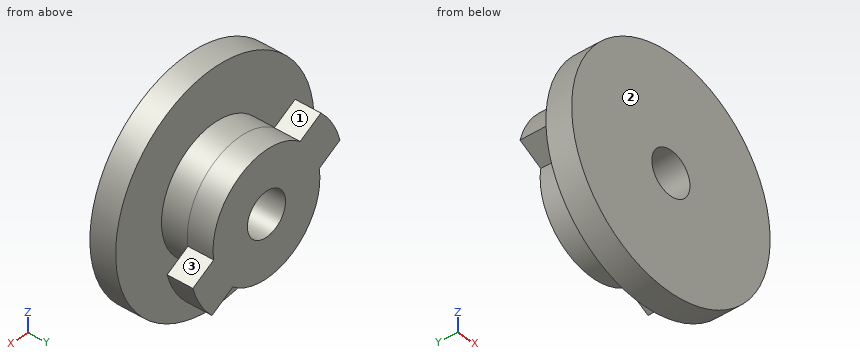
from build123d import *

# Parameters (mm, degrees)
BOSS_EXTRUDE1_DEPTH = 3
BOSS_EXTRUDE2_START = 3
SKETCH2_R           = 7
BOSS_EXTRUDE2_DEPTH = 3
SKETCH3_R           = 13
BOSS_EXTRUDE3_DEPTH = 3
SKETCH4_R           = 2.5
CUT_EXTRUDE1_DEPTH  = 20


with BuildPart() as part:
    # Sketch1 → Boss-Extrude1 (new body)
    with BuildSketch(Plane(origin=(0, 0, 0), x_dir=(-1, 0, 0), z_dir=(0, 1, 0))):
        with BuildLine():
            Line((4.412375826, -57.65977305), (7.135254916, -56.087718075))
            ThreePointArc((7.135254916, -56.087718075), (8.660254038, -58.094010768), (9.635254916, -60.417845094))
            Line((9.635254916, -60.417845094), (6.912375826, -61.989900069))
            ThreePointArc((6.912375826, -61.989900069), (3.5, -69.156188594), (-4.412375826, -68.528248485))
            Line((-4.412375826, -68.528248485), (-7.135254916, -70.10030346))
            ThreePointArc((-7.135254916, -70.10030346), (-8.660254038, -68.094010768), (-9.635254916, -65.770176441))
            Line((-9.635254916, -65.770176441), (-6.912375826, -64.198121466))
            ThreePointArc((-6.912375826, -64.198121466), (-3.5, -57.031832941), (4.412375826, -57.65977305))
        make_face()
    extrude(amount=BOSS_EXTRUDE1_DEPTH)

    # Sketch2 → Boss-Extrude2 (add)
    with BuildSketch(Plane.XZ.offset(BOSS_EXTRUDE2_START)):
        with Locations(Location((0, -63.094010768, 0), (0, 0, 270))):
            Circle(SKETCH2_R)
    extrude(amount=-BOSS_EXTRUDE2_DEPTH)

    # Sketch3 → Boss-Extrude3 (add)
    with BuildSketch(Plane.XZ.offset(3)):
        with Locations(Location((0, -63.094010768, 0), (0, 0, 270))):
            Circle(SKETCH3_R)
    extrude(amount=BOSS_EXTRUDE3_DEPTH)

    # Sketch4 → Cut-Extrude1 (cut)
    with BuildSketch(Plane(origin=(0, 3, 0), x_dir=(1, 0, 0), z_dir=(0, 1, 0))):
        with Locations(Location((0, 63.094010768, 0), (0, 0, 270))):
            Circle(SKETCH4_R)
    extrude(amount=-CUT_EXTRUDE1_DEPTH, mode=Mode.SUBTRACT)


solid = part.part
Work out the finished part from the listing and answer in its coordinate system (mm). Face numbers are marked on the shaded views. Round coordinates to 2 decimals unless told otherwise and drop trailing zeros. Loops run counter-clockwise (first coordinate to the right, second up) from the corner with the lowest first, then second, coordinate; pieces in that order, holes last. Notation, with made-up numbers: (-2, 62) - (17, 62) arc R6 ccw to (17, 66) - close; hole circle Ø9 at (-11.75, 70.5). An arc over 180 degrees is marked (long way). One line per item, written item: value.
Q1. Straight lines are drawn through the part: probe 1 along Y at (x, z) = (-6.5, -57); probe 2 along X at (y, z) = (1.5, -63); probe 3 along Y at (x, z) = (6.75, -70.25). For each, find the intervals that lie inside material, in ascending order.
Check values:
probe 1: -6 to -3, 0 to 3
probe 2: -7 to -2.5, 2.5 to 7
probe 3: -6 to -3
Q2. Find section C-C on y = 1.75. Give the vertices of the cut face in (x, z), and give its area (3 significant figures).
Check values:
outline: (-9.64, -60.42) - (-6.91, -61.99) arc R7 ccw to (4.41, -68.53) - (7.14, -70.1) arc R10 ccw to (9.64, -65.77) - (6.91, -64.2) arc R7 ccw to (-4.41, -57.66) - (-7.14, -56.09) arc R10 ccw to start; hole circle Ø5 at (0, -63.09)
area: 165 mm2
Q3. Find section A-A on x = 0. Give the vertices of the cut face in (y, z), and give its area (3 significant figures).
Check values:
outline: (-6, -76.09) - (-3, -76.09) - (-3, -70.09) - (3, -70.09) - (3, -65.59) - (-6, -65.59) - close; (-6, -60.59) - (3, -60.59) - (3, -56.09) - (-3, -56.09) - (-3, -50.09) - (-6, -50.09) - close
area: 117 mm2
Q4. Each of these flat-tipped pins is pushed along its axis until it touches: pin 1 Ø4 at (x, y) = (-8, 0) entering from +Z; pin 2 Ø2 at (x, y) = (-7, 1.5) entering from -Z. Where does it stop, or does it pass through?
Check values:
pin 1: z = -56.09
pin 2: z = -66.7
Q5. Find section B-B on z = -62.5. Give the vertices of the cut face in (x, y).
Check values:
outline: (-12.99, -6) - (-2.43, -6) - (-2.43, 3) - (-6.97, 3) - (-6.97, -3) - (-12.99, -3) - close; (2.43, -6) - (12.99, -6) - (12.99, -3) - (6.97, -3) - (6.97, 3) - (2.43, 3) - close
Q6. The mould has two halves that part along X. Classify the marked faces 1, 2 and 3: +X half, -X half, draft (parallel to the pull), parting line (faces both ways), or undercut.
Check values:
face 1: undercut
face 2: draft
face 3: +X half
Q7. Find section D-D on x = 9.25. Give the vertices of the cut face in (y, z), and give its area (3 significant figures).
Check values:
outline: (-6, -72.23) - (-3, -72.23) - (-3, -53.96) - (-6, -53.96) - close; (0, -66.89) - (3, -66.89) - (3, -65.55) - (0, -65.55) - close
area: 58.8 mm2
